Source: CAD feature listing. Evaluate the final solid. Frame: model axes, mm. Face numbers are marked on the shaded views. A direction names the side the tool comes from. Give positions to 0.01 mm unless a question says otherwise; leave off trailing zeros. Order: outer loops, then holes, each group sorted by start corner. A loop starts at its lowest first (then second) coordinate and runs counter-clockwise, first axis right, second up. Notation, with made-up numbers: M 84.5,38 L 90.5,38 A25 cw 90.5,70 Z; hole C -25,-28 d10. An arc over 180 degrees is marked long. Answer in a Markdown table with one row per item. Add a question column.
(1) Pin query (flat end, axial travel): P1, Ø6, axis at x = -12, y = 13.5, coming from the -Z side; P2, Ø1, axis at x = 14.5, z = 1, coming from the +Y side; P3, Ø1.1, axis at x = 0, z = 1.5, coming from the +Y side; P4, Ø1.8, axis at y = -7, z = 1.5, coming from the +X side. Return the tip coordinate at first contact, or that it passes through.
(2) Mould query, pull axis X, two halves, no side actions, for the marked faces 1, 2, 3 and 4. Classes: pulls with the +X half, pulls with the -X half, needs draft (parallel to the pull), parting line crosses it, or undercut.
(3) Section query D-D, the plane x = -7. Return loops of the section in (y, z).
(4) Material intervals for line 1 along Y through (x, z) = (2, 0.3); line 2 along X through (y, z) = (-1.5, 2.8); line 3 along X through (y, z) = (-3, 0.95), sorted ascending.
(5) Section query B-B, the plane y = 0. Return loops of the section in (x, z), plus the area to 3 significant figures.
(6) Section query A-A, the plane x = 0. Return loops of the section in (y, z).
(7) Set-up query: the marked faces 5 and 6. Return all of +Z, -Z, +X, -X, +Y, -Y with unobstructed straight access to the full face (end or side cutting, diameter ignored); none if empty.
(8) Section query C-C, the plane z = 3.1. Return loops of the section in (x, y).
Autodesk Inventor part; units mm, degrees
ref_plane "YZ Plane" through (0, 0, 0) normal (1, 0, 0) x (0, 1, 0)
ref_plane "XZ Plane" through (0, 0, 0) normal (0, 1, 0) x (-1, 0, 0)
ref_plane "XY Plane" through (0, 0, 0) normal (0, 0, 1) x (1, 0, 0)
sketch "Sketch1" plane through (0, 0, 0) normal (0, 0, 1) x (1, 0, 0)
  circle A0 centre (0, 0) radius 22
  dimension "d0" = 44
extrude "Extrusion1" add sketch "Sketch1" along normal blind 3.6
sketch "Sketch2" plane through (0, 0, 3.6) normal (0, 0, 1) x (1, 0, 0)
  line L0 (15.3, 0) -> (-15.3, 0) construction
  line L1 (15.3, 5.15) -> (-15.3, 5.15)
  line L2 (-15.3, -5.15) -> (15.3, -5.15)
  arc A0 (15.3, -5.15) -> (15.3, 5.15) centre (15.3, 0) ccw
  arc A1 (-15.3, 5.15) -> (-15.3, -5.15) centre (-15.3, 0) ccw
  point P0 (0, 0)
  dimension "d3" = 15.3
  dimension "d4" = 10.3
extrude "Extrusion2" cut sketch "Sketch2" against normal blind 3.6
sketch "Sketch3" plane through (0, 0, 3.6) normal (0, 0, 1) x (1, 0, 0)
  line L0 (-2.6, 9.8) -> (2.6, 9.8)
  line L1 (2.6, 9.8) -> (2.6, 6)
  line L2 (2.6, 6) -> (-2.6, 6)
  line L3 (-2.6, 6) -> (-2.6, 9.8)
  line L4 (-2.6, 9.8) -> (2.6, 6) construction
  line L5 (2.6, 9.8) -> (-2.6, 6) construction
  line L6 (-30.8, 0) -> (30.8, 0)
  line L7 (-30.8, 0) -> (30.8, 0)
  line L8 (-2.6, -9.8) -> (2.6, -9.8)
  line L9 (2.6, -9.8) -> (2.6, -6)
  line L10 (2.6, -6) -> (-2.6, -6)
  line L11 (-2.6, -6) -> (-2.6, -9.8)
  line L12 (-2.6, -9.8) -> (2.6, -6) construction
  line L13 (2.6, -9.8) -> (-2.6, -6) construction
  point P0 (0, 0)
  point P1 (0, 7.9)
  point P2 (0, -7.9)
  dimension "d7" = 5.2
  dimension "d8" = 3.8
  dimension "d9" = 6
  dimension "d10" = 6
  dimension "d13" = 0
extrude "Extrusion3" cut sketch "Sketch3" against normal blind 10
properties part number "1"
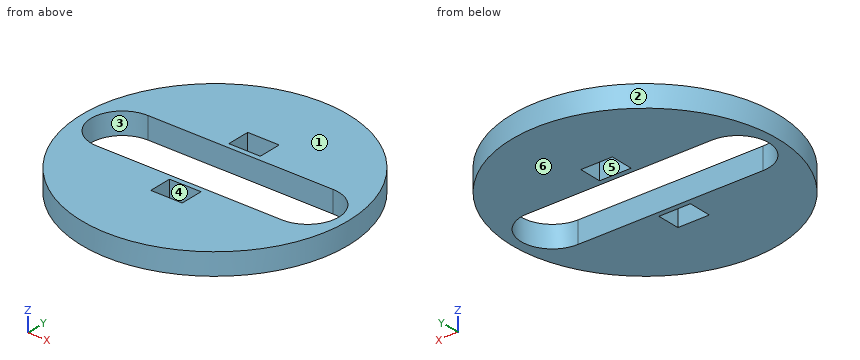
Values follow:
| question | item | result |
|---|---|---|
| 1 | P1 | stops at z = 0 |
| 1 | P2 | stops at y = 16.97 |
| 1 | P3 | stops at y = 22 |
| 1 | P4 | stops at x = 21.14 |
| 2 | face 1 | needs draft |
| 2 | face 2 | parting line crosses it |
| 2 | face 3 | undercut |
| 2 | face 4 | undercut |
| 3 | outline | M -20.86,0 L -5.15,0 L -5.15,3.6 L -20.86,3.6 Z; M 5.15,0 L 20.86,0 L 20.86,3.6 L 5.15,3.6 Z |
| 4 | line 1 | y = -21.91 to -9.8, -6 to -5.15, 5.15 to 6, 9.8 to 21.91 |
| 4 | line 2 | x = -21.95 to -20.23, 20.23 to 21.95 |
| 4 | line 3 | x = -21.79 to -19.49, 19.49 to 21.79 |
| 5 | outline | M -22,0 L -20.45,0 L -20.45,3.6 L -22,3.6 Z; M 20.45,0 L 22,0 L 22,3.6 L 20.45,3.6 Z |
| 5 | area | 11.2 mm² |
| 6 | outline | M -22,0 L -9.8,0 L -9.8,3.6 L -22,3.6 Z; M -6,0 L -5.15,0 L -5.15,3.6 L -6,3.6 Z; M 5.15,0 L 6,0 L 6,3.6 L 5.15,3.6 Z; M 9.8,0 L 22,0 L 22,3.6 L 9.8,3.6 Z |
| 7 | face 5 | +Z, -Z |
| 7 | face 6 | -Z, +X, -X, +Y, -Y |
| 8 | outline | C 0,0 d44; hole M -15.3,-5.15 L 15.3,-5.15 A5.15 ccw 15.3,5.15 L -15.3,5.15 A5.15 ccw Z; hole M -2.6,-9.8 L 2.6,-9.8 L 2.6,-6 L -2.6,-6 Z; hole M -2.6,6 L 2.6,6 L 2.6,9.8 L -2.6,9.8 Z |
